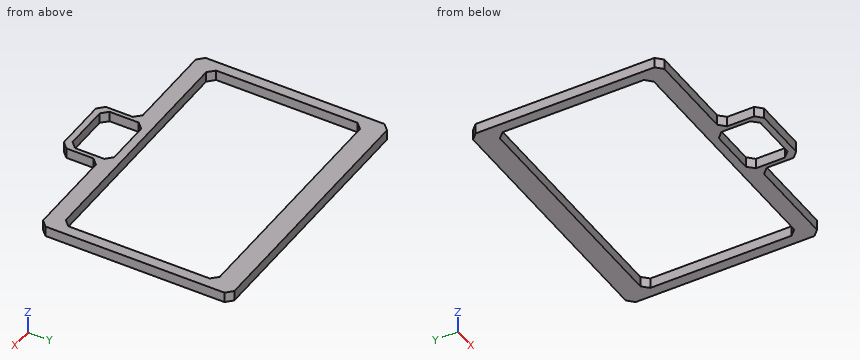
```python
from build123d import *

# Parameters (mm, degrees)
BOSS_EXTRUDE1_DEPTH = 5


with BuildPart() as part:
    # Sketch1 → Boss-Extrude1 (new body)
    with BuildSketch(Plane.XY):
        Polygon((3, 10), (127, 10), (130, 7), (130, -79), (127, -82), (84, -82), (81, -85), (81, -98), (78, -101), (52, -101), (49, -98), (49, -85), (46, -82), (3, -82), (0, -79), (0, 7), align=None)
        Polygon((125, -71), (125, -3), (122, 0), (8, 0), (5, -3), (5, -71), (8, -74), (122, -74), align=None, mode=Mode.SUBTRACT)
        Polygon((54, -78), (76, -78), (79, -81), (79, -95), (76, -98), (54, -98), (51, -95), (51, -81), align=None, mode=Mode.SUBTRACT)
    extrude(amount=BOSS_EXTRUDE1_DEPTH)


solid = part.part
```
The model under review builds one solid part; all positions refer to its coordinate system, in mm. Round coordinates to 2 decimals unless told otherwise and drop trailing zeros. Loops run counter-clockwise (first coordinate to the right, second up) from the corner with the lowest first, then second, coordinate; pieces in that order, holes last.
Item 1: Take a section at A-A (x = 86.5). Write out the cut boundary in (y, z), then the cut area to 3 significant figures.
Determined:
outline: (-82, 0) - (-74, 0) - (-74, 5) - (-82, 5) - close; (0, 0) - (10, 0) - (10, 5) - (0, 5) - close
area: 90.0 mm2
Item 2: For line 1 (X direction, y = -10, z = 4.6); line 2 (Y direction, x = 96, z = 2.25); line 3 (X direction, y = -85, z = 3.15), list the stretches that pass through material, from the lowest coordinate up.
Determined:
line 1: x = 0 to 5, 125 to 130
line 2: y = -82 to -74, 0 to 10
line 3: x = 49 to 51, 79 to 81
Item 3: Clearance check with flat-ended pins moving along their axes: pin 1 Ø1.5 at (x, z) = (24.5, 3.5) entering from -Y; pin 2 Ø1.5 at (y, z) = (-92.5, 1.5) entering from +X. State where each tip first meets the part, or that it passes through.
Determined:
pin 1: stops at y = -82
pin 2: stops at x = 81
Item 4: Take a section at B-B (z = 1.45). Give the number of separate pieces and of enclosed holes in the cut face, then the cut area to 3 significant figures.
Determined:
separate pieces: 1
enclosed holes: 2
area: 3,150 mm2
Item 5: Take a section at D-D (x = 73.5). Write out the cut boundary in (y, z).
Determined:
outline: (-101, 0) - (-98, 0) - (-98, 5) - (-101, 5) - close; (-78, 0) - (-74, 0) - (-74, 5) - (-78, 5) - close; (0, 0) - (10, 0) - (10, 5) - (0, 5) - close
Item 6: Take a section at C-C (y = -87). Write out the cut boundary in (x, z), then the cut area to 3 significant figures.
Determined:
outline: (49, 0) - (51, 0) - (51, 5) - (49, 5) - close; (79, 0) - (81, 0) - (81, 5) - (79, 5) - close
area: 20.0 mm2
